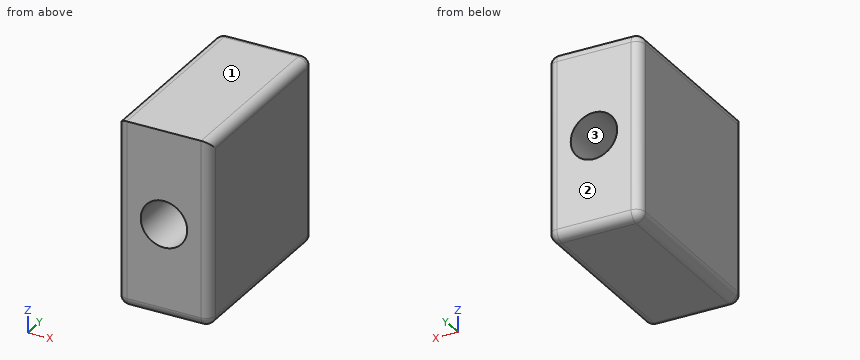
```python
from build123d import *

# Parameters (mm, degrees)
F0_W     = 50.8
F0_H     = 101.6
F1_DEPTH = 101.6
F2_R     = 12.7
F3_DEPTH = 101.6
F4_R     = 5.08


with BuildPart() as f1:
    # F0 (on Front) → F1 (new body)
    with BuildSketch(Plane.XZ):
        Rectangle(F0_W, F0_H)
    extrude(amount=-F1_DEPTH)

    # F2 (on Front) → F3 (cut, through all)
    with BuildSketch(Plane.XZ):
        Circle(F2_R)
    extrude(amount=-F3_DEPTH, mode=Mode.SUBTRACT)

    # F4
    f4_edges = [f1.edges().sort_by_distance(p)[0] for p in [
        (25.4, 50.8, 50.8),
        (-25.4, 50.8, 50.8),
        (25.4, 50.8, -50.8),
        (-25.4, 50.8, -50.8),
        (0, 101.6, -50.8),
        (-25.4, 101.6, 0),
        (0, 101.6, 50.8),
        (25.4, 101.6, 0),
        (25.4, 0, 0),
        (-25.4, 0, 0),
        (0, 0, -50.8),
    ]]
    fillet(f4_edges, radius=F4_R)


solid = f1.part
```
Can you work these out from the model? Positions are in its coordinate system, mm. Face numbers are marked on the shaded views. Round coordinates to 2 decimals unless told otherwise and drop trailing zeros. Loops run counter-clockwise (first coordinate to the right, second up) from the corner with the lowest first, then second, coordinate; pieces in that order, holes last. Notation, with made-up numbers: M 52,-32 L 70,-32 A22 ccw 70,-14 Z; hole C -12.75,-21 d2. An arc over 180 degrees is marked long. Answer as a JSON object with one key per item and string values. Group by question number.
Q1. Imagine slicing it at A-A, the plane x = 0. Please give me the cut outline in (y, z), then the cut area to 3 significant figures.
Q2. Imagine slicing it at D-D, the plane x = 6. Please give me the cut outline in (y, z).
Q3. Imagine slicing it at C-C, the plane y = 59. Please give me the cut outline in (x, z), then the cut area to 3 significant figures.
Q4. Imagine slicing it at B-B, the plane z = 8.5. Please give me the cut outline in (x, y), then the cut area to 3 significant figures.
Q5. We'd pull the mould along Z, two halves only. Please class the marked faces 1, 2 and 3: +Z half, -Z half, draft (parallel to the pull), parting line (faces both ways), or undercut.
Q6. Please list where these lines run through material, in increasing order: L1, parallel to Z at x = 0.5, y = 42.5; L2, parallel to X at y = 92, z = 10.5; L3, parallel to X at y = 25, z = -9.
Findings:
{
 "1": {"outline": "M 0,-45.72 A5.08 ccw 5.08,-50.8 L 96.52,-50.8 A5.08 ccw 101.6,-45.72 L 101.6,-12.7 L 0,-12.7 Z; M 0,12.7 L 101.6,12.7 L 101.6,45.72 A5.08 ccw 96.52,50.8 L 0,50.8 Z", "area": "7,730 mm2"},
 "2": {"outline": "M 0,-45.72 A5.08 ccw 5.08,-50.8 L 96.52,-50.8 A5.08 ccw 101.6,-45.72 L 101.6,-11.19 L 0,-11.19 Z; M 0,11.19 L 101.6,11.19 L 101.6,45.72 A5.08 ccw 96.52,50.8 L 0,50.8 Z"},
 "3": {"outline": "M -25.4,-45.72 A5.08 ccw -20.32,-50.8 L 20.32,-50.8 A5.08 ccw 25.4,-45.72 L 25.4,45.72 A5.08 ccw 20.32,50.8 L -20.32,50.8 A5.08 ccw -25.4,45.72 Z; hole C 0,0 d25.4", "area": "4,630 mm2"},
 "4": {"outline": "M -25.4,5.08 A5.08 ccw -20.32,0 L -9.44,0 L -9.44,101.6 L -20.32,101.6 A5.08 ccw -25.4,96.52 Z; M 9.44,0 L 20.32,0 A5.08 ccw 25.4,5.08 L 25.4,96.52 A5.08 ccw 20.32,101.6 L 9.44,101.6 Z", "area": "3,220 mm2"},
 "5": {"face 1": "+Z half", "face 2": "draft", "face 3": "undercut"},
 "6": {"L1": "z = -50.8 to -12.69, 12.69 to 50.8", "L2": "x = -25.4 to -7.14, 7.14 to 25.4", "L3": "x = -25.4 to -8.96, 8.96 to 25.4"}
}
